from build123d import *

# Parameters (mm, degrees)
ESQUISSE2_R                  = 10
ENL_V_MAT_EXTRU_1_DEPTH      = 687.62944883
R_P_TITION_CIRCULAIRE1_COUNT = 20


with BuildPart() as part:
    # Esquisse1 → Révolution1 (revolve)
    with BuildSketch(Plane.XY, mode=Mode.PRIVATE) as r_volution1_sk:
        with BuildLine():
            Line((0, 0), (80, 0))
            Line((80, 0), (80, 52.5))
            ThreePointArc((80, 52.5), (70, 62.5), (80, 72.5))
            Line((80, 72.5), (80, 90))
            Line((80, 90), (0, 90))
            Line((0, 90), (0, 0))
        make_face()
    revolve(r_volution1_sk.sketch.rotate(Axis((-256, 27.419354839, 0), (0, -1, 0)), 90), axis=Axis((-256, 27.419354839, 0), (0, -1, 0)))

    # Esquisse2 → Enlèv. mat.-Extru.1 (cut, through all)
    with BuildSketch(Plane.XZ):
        with Locations(Location((40, 0, 0), (0, 0, 270))):
            Circle(ESQUISSE2_R)
    enl_v_mat_extru_1 = extrude(amount=-ENL_V_MAT_EXTRU_1_DEPTH, mode=Mode.SUBTRACT)

    # Répétition circulaire1: Enlèv. mat.-Extru.1 ×20 about axis
    r_p_tition_circulaire1_axis = Axis((-256, 0, 0), (0, 1, 0))
    for i in range(1, R_P_TITION_CIRCULAIRE1_COUNT):
        add(enl_v_mat_extru_1.rotate(r_p_tition_circulaire1_axis, i * 360 / R_P_TITION_CIRCULAIRE1_COUNT), mode=Mode.SUBTRACT)


solid = part.part
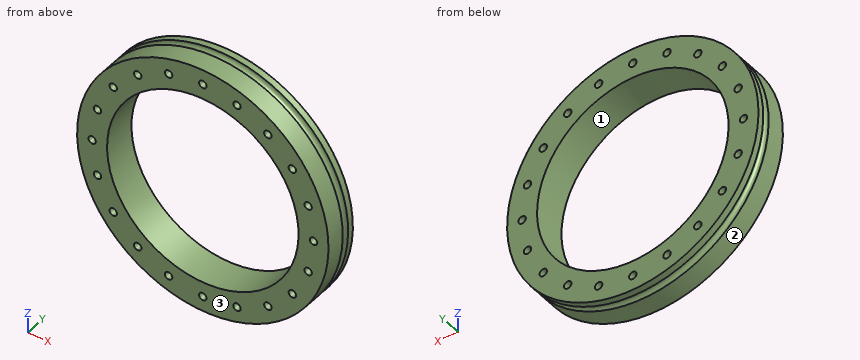
Can you work these out from the model? Positions are in its coordinate system, mm. Face numbers are marked on the shaded views. Coordinates: 2 decimals unless noted, no trailing zeros. Write each loop counter-clockwise with the first axis right and the second up, starting at its lowest first coordinate (ties: lowest second). Pieces come first, ordered by that corner, then holes. Notation, with made-up numbers: M 81.25,56 L 103.25,56 A33 cw 103.25,91 Z; hole C 5.5,87.5 d4. An arc over 180 degrees is marked long. Use one line per item in the form item = value.
Q1. We'd pull the mould along X, two halves only. Please class the marked faces 1, 2 and 3: +X half, -X half, draft (parallel to the pull), parting line (faces both ways), or undercut.
Model answer:
face_1 = undercut
face_2 = parting line
face_3 = draft
Q2. If we section it at A-A (x = -256): Write out the boundary of the cut face in (y, z).
Model answer:
outline = M 0,-336 L 52.5,-336 A10 cw 72.5,-336 L 90,-336 L 90,-306 L 0,-306 Z; M 0,-286 L 90,-286 L 90,-256 L 0,-256 Z; M 0,256 L 90,256 L 90,286 L 0,286 Z; M 0,306 L 90,306 L 90,336 L 72.5,336 A10 cw 52.5,336 L 0,336 Z
Q3. If we section it at C-C (y = 34.5): State how many separate pieces and enclosed holes the cut face has, then the cut area to 3 significant figures.
Model answer:
separate_pieces = 1
enclosed_holes = 21
area = 143,000 mm^2
Q4. If we section it at B-B (z = 0): Write out the boundary of the cut face in (x, y), then the cut area to 3 significant figures.
Model answer:
outline = M -592,0 L -562,0 L -562,90 L -592,90 L -592,72.5 A10 cw -592,52.5 Z; M -542,0 L -512,0 L -512,90 L -542,90 Z; M 0,0 L 30,0 L 30,90 L 0,90 Z; M 50,0 L 80,0 L 80,52.5 A10 cw 80,72.5 L 80,90 L 50,90 Z
area = 10,500 mm^2
Q5. I need wall thicknesses on line 1 along X through (y, z) = (49, -168.5); line 2 along Z through (x, y) = (-169, 12.5); line 3 along X through (y, z) = (26, -178). Which ranges of each line are inside material? Lowest first, please. Write a range as from..to.
Model answer:
line_1 = -546.7..-503.83, -487.11..-448.73, -63.27..-24.89, -8.17..34.7
line_2 = -324.54..-290.46, -272.57..-240.76, 240.76..272.57, 290.46..324.54
line_3 = -540.98..-504.63, -486.31..-439.99, -72.01..-25.69, -7.37..28.98
Q6. For P1, Ø10, axis at y = 70, z = 46, coming from the +X side; P2, Ø12, axis at x = -41.5, y = 46, coming from the -Z side; P3, Ø8, axis at y = 74, z = -30, coming from the -X side, each with a flat end and sliding along its axis, tell me the tip position at first contact or that it passes through.
Model answer:
P1 = 77.41
P2 = -263.48
P3 = -590.99
